Design review of the part built by this model. Coordinates are the model's own, in mm. Coordinates: 2 decimals unless noted, no trailing zeros. Loops run counter-clockwise (first coordinate to the right, second up) from the corner with the lowest first, then second, coordinate; pieces in that order, holes last.
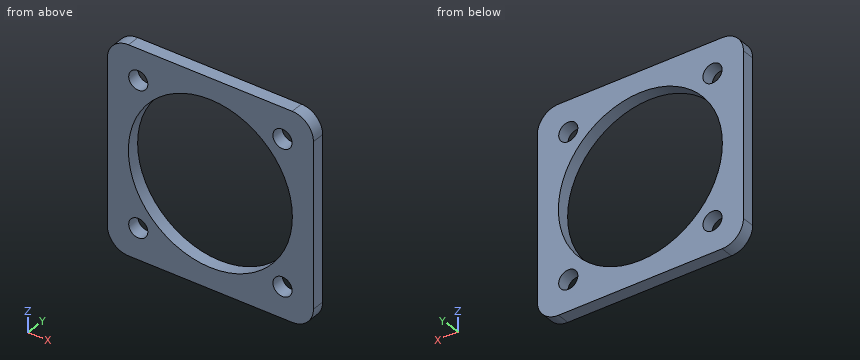
from build123d import *

# Parameters (mm, degrees)
SKETCH_1_R      = 19.3
SKETCH_1_R_2    = 2.25
EXTRUDE_1_DEPTH = 3


with BuildPart() as part:
    # 草图1 → 凸台-拉伸1 (new body)
    with BuildSketch(Plane(origin=(0, 0, 0), x_dir=(1, 0, 0), z_dir=(0, 1, 0))):
        with BuildLine():
            Line((-19.253762595, -24.253762595), (19.253762595, -24.253762595))
            ThreePointArc((19.253762595, -24.253762595), (22.789296501, -22.789296501), (24.253762595, -19.253762595))
            Line((24.253762595, -19.253762595), (24.253762595, 19.253762595))
            ThreePointArc((24.253762595, 19.253762595), (22.789296501, 22.789296501), (19.253762595, 24.253762595))
            Line((19.253762595, 24.253762595), (-19.253762595, 24.253762595))
            ThreePointArc((-19.253762595, 24.253762595), (-22.789296501, 22.789296501), (-24.253762595, 19.253762595))
            Line((-24.253762595, 19.253762595), (-24.253762595, -19.253762595))
            ThreePointArc((-24.253762595, -19.253762595), (-22.789296501, -22.789296501), (-19.253762595, -24.253762595))
        make_face()
        with Locations(Location((0, 0, 0), (0, 0, 270))):
            Circle(SKETCH_1_R, mode=Mode.SUBTRACT)
        with Locations(Location((-16.970562748, 16.970562748, 0), (0, 0, 270))):
            Circle(SKETCH_1_R_2, mode=Mode.SUBTRACT)
        with Locations(Location((16.970562748, 16.970562748, 0), (0, 0, 270))):
            Circle(SKETCH_1_R_2, mode=Mode.SUBTRACT)
        with Locations(Location((16.970562748, -16.970562748, 0), (0, 0, 270))):
            Circle(SKETCH_1_R_2, mode=Mode.SUBTRACT)
        with Locations(Location((-16.970562748, -16.970562748, 0), (0, 0, 270))):
            Circle(SKETCH_1_R_2, mode=Mode.SUBTRACT)
    extrude(amount=EXTRUDE_1_DEPTH)


solid = part.part
Q1. Take a section at C-C, the plane z = 17.5. Write out the cut boundary in (x, y), then the cut area to 3 significant figures.
Q2. Take a section at A-A, the plane z = 0. Write out the cut boundary in (x, y), then the cut area to 3 significant figures.
Q3. Take a section at D-D, the plane y = 0.7. Write out the cut boundary in (x, z), then the cut area to 3 significant figures.
Q4. For line 1 (X direction, y = 1.6, z = 0); line 2 (Z direction, x = 1.5, y = 2.2); line 3 (Z direction, x = -15.5, y = 0.3), list the stretches that pass through material, from the lowest coordinate up.
Q5. Take a section at B-B, the plane x = 0. Write out the cut boundary in (y, z), then the cut area to 3 significant figures.
Q6. Clearance check with a flat-ended pin moving along its axis: pin 1 Ø6 at (x, z) = (16.97, -16.97) entering from +Y. State where the tip first meets the part, or that it passes through.
Entries:
1. outline: (-24.25, 0) - (-19.16, 0) - (-19.16, 3) - (-24.25, 3) - close; (-14.78, 0) - (-8.14, 0) - (-8.14, 3) - (-14.78, 3) - close; (8.14, 0) - (14.78, 0) - (14.78, 3) - (8.14, 3) - close; (19.16, 0) - (24.25, 0) - (24.25, 3) - (19.16, 3) - close
1. area: 70.4 mm2
2. outline: (-24.25, 0) - (-19.3, 0) - (-19.3, 3) - (-24.25, 3) - close; (19.3, 0) - (24.25, 0) - (24.25, 3) - (19.3, 3) - close
2. area: 29.7 mm2
3. outline: (-24.25, -19.25) arc R5 ccw to (-19.25, -24.25) - (19.25, -24.25) arc R5 ccw to (24.25, -19.25) - (24.25, 19.25) arc R5 ccw to (19.25, 24.25) - (-19.25, 24.25) arc R5 ccw to (-24.25, 19.25) - close; hole circle Ø38.6 at (0, 0); hole circle Ø4.5 at (-16.97, -16.97); hole circle Ø4.5 at (-16.97, 16.97); hole circle Ø4.5 at (16.97, -16.97); hole circle Ø4.5 at (16.97, 16.97)
3. area: 1,100 mm2
4. line 1: x = -24.25 to -19.3, 19.3 to 24.25
4. line 2: z = -24.25 to -19.24, 19.24 to 24.25
4. line 3: z = -24.25 to -18.67, -15.27 to -11.5, 11.5 to 15.27, 18.67 to 24.25
5. outline: (0, -24.25) - (3, -24.25) - (3, -19.3) - (0, -19.3) - close; (0, 19.3) - (3, 19.3) - (3, 24.25) - (0, 24.25) - close
5. area: 29.7 mm2
6. pin 1: stops at y = 3
